The listing builds one solid part. Answer for the finished solid, in the listing's coordinates (mm). A direction names the side the tool comes from. Coordinates: 2 decimals unless noted, no trailing zeros. Loops run counter-clockwise (first coordinate to the right, second up) from the corner with the lowest first, then second, coordinate; pieces in that order, holes last. Notation, with made-up numbers: M 15,-20 L 65,-20 A20 cw 65,18 Z; hole C -17,66.5 d3. An arc over 180 degrees is marked long. Return JSON: item names as keys, results as strings. Group by question number.
1. Given P1, Ø6.5, axis at x = 19, z = 4, coming from the +Y side; P2, Ø5, axis at x = 19, z = -4, coming from the -Y side; P3, Ø4.5, axis at x = 19, z = -3.5, coming from the +Y side; P4, Ø2.5, axis at x = -19, z = 4, coming from the +Y side, each flat-ended and moving along its own axis, determine where each tip first touches the part or whether it passes through.
2. Straight lines are drawn through the part: L1, parallel to X at y = 19.45, z = -4; L2, parallel to Z at x = 19, y = 20; L3, parallel to Y at x = -15.5, z = 1.25. For each, find the intervals that lie inside material, in ascending order. Write a range as from..to.
3. Section B-B (x = 19) is taken. Write down the section's boundary in (y, z), then the cut area to 4 significant figures.
4. Section D-D (z = 0) is taken. Write down the section's boundary in (x, y).
5. Which of the six approach directions +Z, -Z, +X, -X, +Y, -Y give full straight-line access (tool end or side, diameter ignored) to faces 1 (the face through (19, 21, 0)), 2 (the face through (-15.9, 9, 0)), 3 (the face through (-10.1, 30, -1.2)), 4 (the face through (-15.9, 25, 0))?
6. The mould has two halves that part along X. Classify faces 5 (the face through (-5.55, 31.48, -0.72)), 6 (the face through (-17.06, 19.77, 4.8)), 7 (the face through (-19, 18.5, 0)): pulls with the +X half, pulls with the -X half, needs draft (parallel to the pull), parting line crosses it, or undercut.
7. Section C-C (y = 20) is taken. Write down the section's boundary in (x, z).
8. Section A-A (z = 4) is taken. Write down the section's boundary in (x, y).
```python
from build123d import *

# Parameters (mm, degrees)
SKETCH1_W           = 31.8
SKETCH1_H           = 16.5
BOSS_EXTRUDE1_DEPTH = 28.4
SKETCH2_W           = 16.5
SKETCH2_H           = 2.5
BOSS_EXTRUDE2_DEPTH = 5.5
SKETCH3_R           = 2.1
CUT_EXTRUDE1_DEPTH  = 2.5
SKETCH4_R           = 5
BOSS_EXTRUDE3_DEPTH = 1.6
SKETCH5_R           = 2.4
BOSS_EXTRUDE4_DEPTH = 3
CHAMFER1_SIZE       = 5
CHAMFER1_SIZE2      = 7.140740034


with BuildPart() as part:
    # Sketch1 → Boss-Extrude1 (new body)
    with BuildSketch(Plane(origin=(0, 0, 0), x_dir=(1, 0, 0), z_dir=(0, 1, 0))):
        Rectangle(SKETCH1_W, SKETCH1_H)
    extrude(amount=BOSS_EXTRUDE1_DEPTH)

    # Sketch2 → Boss-Extrude2 (add)
    with BuildSketch(Plane(origin=(15.9, 0, 0), x_dir=(0, 0, -1), z_dir=(1, 0, 0))):
        with Locations((0, 19.75)):
            Rectangle(SKETCH2_W, SKETCH2_H)
    boss_extrude2 = extrude(amount=BOSS_EXTRUDE2_DEPTH)

    # Mirror1: Boss-Extrude2 across plane
    add(boss_extrude2.mirror(Plane(origin=(0, 0, 0), x_dir=(0, 0, 1), z_dir=(1, 0, 0))))

    # Sketch3 → Cut-Extrude1 (cut)
    with BuildSketch(Plane(origin=(0, 21, 0), x_dir=(1, 0, 0), z_dir=(0, 1, 0))):
        with Locations((-19, 4)):
            Circle(SKETCH3_R)
        with Locations((-19, -4)):
            Circle(SKETCH3_R)
        with Locations((19, 4)):
            Circle(SKETCH3_R)
        with Locations((19, -4)):
            Circle(SKETCH3_R)
    extrude(amount=-CUT_EXTRUDE1_DEPTH, mode=Mode.SUBTRACT)

    # Sketch4 → Boss-Extrude3 (add)
    with BuildSketch(Plane(origin=(0, 28.4, 0), x_dir=(1, 0, 0), z_dir=(0, 1, 0))):
        with Locations((-7.84, 0)):
            Circle(SKETCH4_R)
    extrude(amount=BOSS_EXTRUDE3_DEPTH)

    # Sketch5 → Boss-Extrude4 (add)
    with BuildSketch(Plane(origin=(0, 30, 0), x_dir=(1, 0, 0), z_dir=(0, 1, 0))):
        with Locations((-7.84, 0)):
            Circle(SKETCH5_R)
    extrude(amount=BOSS_EXTRUDE4_DEPTH)

    # Chamfer1
    chamfer1_edges = [part.edges().sort_by_distance(p)[0] for p in [
        (15.9, 28.4, 0),
    ]]
    chamfer1_side = [part.faces().sort_by_distance(p)[0] for p in [
        (15.9, 24.7, 0),
    ]]
    chamfer(chamfer1_edges, length=CHAMFER1_SIZE, length2=CHAMFER1_SIZE2, reference=chamfer1_side[0])


solid = part.part
```
Worked out:
{
 "1": {"P1": "y = 23.51", "P2": "y = 18.5", "P3": "y = 21", "P4": "through"},
 "2": {"L1": "-21.4..-21.1, -16.9..16.9, 21.1..21.4", "L2": "-8.25..-6.1, -1.9..1.9, 6.1..8.25", "L3": "0..28.4"},
 "3": {"outline": "M 18.5,-8.25 L 21,-8.25 L 21,-6.1 L 18.5,-6.1 Z; M 18.5,-1.9 L 21,-1.9 L 21,1.9 L 18.5,1.9 Z; M 18.5,6.1 L 21,6.1 L 21,8.25 L 18.5,8.25 Z", "area": "20.25 mm^2"},
 "4": {"outline": "M -21.4,18.5 L -15.9,18.5 L -15.9,0 L 15.9,0 L 15.9,18.5 L 21.4,18.5 L 21.4,21 L 15.9,21 L 15.9,23.4 L 8.76,28.4 L -2.84,28.4 L -2.84,30 L -5.44,30 L -5.44,33 L -10.24,33 L -10.24,30 L -12.84,30 L -12.84,28.4 L -15.9,28.4 L -15.9,21 L -21.4,21 Z"},
 "5": {"face 1": "+Z, -Z, +X, +Y", "face 2": "+Z, -Z, -X, -Y", "face 3": "+Y", "face 4": "+Z, -Z, -X, +Y"},
 "6": {"face 5": "parting line crosses it", "face 6": "undercut", "face 7": "needs draft"},
 "7": {"outline": "M -21.4,-8.25 L 21.4,-8.25 L 21.4,8.25 L -21.4,8.25 Z; hole C -19,-4 d4.2; hole C -19,4 d4.2; hole C 19,-4 d4.2; hole C 19,4 d4.2"},
 "8": {"outline": "M -21.4,18.5 L -21.1,18.5 L -21.1,21 L -21.4,21 Z; M -16.9,18.5 L -15.9,18.5 L -15.9,0 L 15.9,0 L 15.9,18.5 L 16.9,18.5 L 16.9,21 L 15.9,21 L 15.9,23.4 L 8.76,28.4 L -4.84,28.4 L -4.84,30 L -10.84,30 L -10.84,28.4 L -15.9,28.4 L -15.9,21 L -16.9,21 Z; M 21.1,18.5 L 21.4,18.5 L 21.4,21 L 21.1,21 Z"}
}
